```python
from build123d import *

# Parameters (mm, degrees)
SKETCH_1_W          = 10
SKETCH_1_H          = 20
SKETCH_1_W_2        = 7.6
SKETCH_1_H_2        = 17.6
EXTRUDE_1_DEPTH     = 379.5
SKETCH_2_R          = 2
CUT_EXTRUDE_1_DEPTH = 381.05953481
SKETCH_3_R          = 2
CUT_EXTRUDE_2_DEPTH = 380.763413193


with BuildPart() as part:
    # ｽｹｯﾁ1 → 押し出し-薄板1 (new body)
    with BuildSketch(Plane.XY):
        Rectangle(SKETCH_1_W, SKETCH_1_H)
        Rectangle(SKETCH_1_W_2, SKETCH_1_H_2, mode=Mode.SUBTRACT)
    extrude(amount=EXTRUDE_1_DEPTH)

    # ｽｹｯﾁ2 → ｶｯﾄ - 押し出し1 (cut, through all)
    with BuildSketch(Plane(origin=(0, 10, 0), x_dir=(1, 0, 0), z_dir=(0, 1, 0))):
        with Locations(Location((0, -364.5, 0), (0, 0, 270))):
            Circle(SKETCH_2_R)
        with Locations(Location((0, -374.5, 0), (0, 0, 270))):
            Circle(SKETCH_2_R)
        with Locations(Location((0, -244.5, 0), (0, 0, 270))):
            Circle(SKETCH_2_R)
        with Locations(Location((0, -120, 0), (0, 0, 270))):
            Circle(SKETCH_2_R)
        with Locations(Location((0, -20, 0), (0, 0, 270))):
            Circle(SKETCH_2_R)
    extrude(amount=-CUT_EXTRUDE_1_DEPTH, mode=Mode.SUBTRACT)

    # ｽｹｯﾁ3 → ｶｯﾄ - 押し出し2 (cut, through all)
    with BuildSketch(Plane(origin=(5, 0, 0), x_dir=(0, 0, -1), z_dir=(1, 0, 0))):
        with Locations(Location((-7.5, 5, 0), (0, 0, 90))):
            Circle(SKETCH_3_R)
        with Locations(Location((-7.5, -5, 0), (0, 0, 90))):
            Circle(SKETCH_3_R)
        with Locations(Location((-70, 0, 0), (0, 0, 90))):
            Circle(SKETCH_3_R)
        with Locations(Location((-50, 0, 0), (0, 0, 90))):
            Circle(SKETCH_3_R)
    extrude(amount=-CUT_EXTRUDE_2_DEPTH, mode=Mode.SUBTRACT)


solid = part.part
```
Geometry check sheet. Reference: the model listing, model coordinates, mm. A direction names the side the tool comes from. Round coordinates to 2 decimals unless told otherwise and drop trailing zeros. Loops run counter-clockwise (first coordinate to the right, second up) from the corner with the lowest first, then second, coordinate; pieces in that order, holes last. Notation, with made-up numbers: M -17.5,-20.5 L 32.5,-20.5 A6 ccw 32.5,-14.5 Z; hole C 86.5,-38.5 d2. An arc over 180 degrees is marked long. Return JSON: item names as keys, results as strings. Group by question number.
(1) Scan lines: line 1 along Z through (x, y) = (-4.5, 0); line 2 along Z through (x, y) = (-4.7, -5); line 3 along X through (y, z) = (9.7, 120). Record each from-to range of solid material in increasing order. Write a range as [from, to].
(2) Go/stop test with a flat-tipped pin: pin 1 (3.5 mm diameter, centred on x = 0, z = 120, fed in from +Y). Record where the tip stops, or that it passes through.
(3) Set-up check for faces 1 (the face through (-4, -1, 379.5)), 2 (the face through (0, -8.8, 187)): record each of +Z, -Z, +X, -X, +Y, -Y from which the full face is reachable in a straight line by a thin tool's end or side.
(4) Section check A-A, the plane z = 321. Enter the section's corners in (x, y), and give its area (3 significant figures).
(5) Mould release check, pull along Y, two halves, no side actions. Record for faces 3 (the face through (0, 10, 187)), 4 (the face through (0, -10, 187)), 5 (the face through (-3.8, 0, 187)): pulls with the +Y half, pulls with the -Y half, needs draft (parallel to the pull), parting line crosses it, or undercut.
Data:
{
 "1": {"line 1": "[0, 48], [52, 68], [72, 379.5]", "line 2": "[0, 5.5], [9.5, 379.5]", "line 3": "[-5, -2], [2, 5]"},
 "2": {"pin 1": "through"},
 "3": {"face 1": "+Z, +X, -X, +Y, -Y", "face 2": "+Z, -Z"},
 "4": {"outline": "M -5,-10 L 5,-10 L 5,10 L -5,10 Z; hole M -3.8,-8.8 L 3.8,-8.8 L 3.8,8.8 L -3.8,8.8 Z", "area": "66.2 mm²"},
 "5": {"face 3": "pulls with the +Y half", "face 4": "pulls with the -Y half", "face 5": "undercut"}
}
